Autodesk Inventor part; units mm, degrees
ref_plane "Work Plane5" through (0, -10, 0) normal (0, 1, 0) x (-1, 0, 0)
ref_plane "YZ Plane" through (0, 0, 0) normal (1, 0, 0) x (0, 1, 0)
ref_plane "XY Plane" through (0, 0, 0) normal (0, 0, 1) x (1, 0, 0)
sketch "Sketch1" plane through (0, 0, 0) normal (0, 0, 1) x (1, 0, 0)
  line L0 (-3.9007, 3.9007) -> (3.9007, 3.9007)
  line L1 (3.9007, 3.9007) -> (3.9007, -3.9007)
  line L2 (3.9007, -3.9007) -> (-3.9007, -3.9007)
  line L3 (-3.9007, -3.9007) -> (-3.9007, 3.9007)
  line L4 (0, 3.9007) -> (0, -3.9007) construction
  line L5 (-3.9007, 0) -> (3.9007, 0) construction
  circle A0 centre (0, 0) radius 2.1
  line L6 (0, 0) -> (-16.1173, 16.1173) construction
  line L7 (0, 0) -> (22.7933, 0) construction
  line L8 (-2.84, 3.9007) -> (-5.4993, 6.56)
  line L9 (-5.4993, 6.56) -> (-5.4993, 8.2)
  line L10 (-5.4993, 8.2) -> (-2.84, 8.2)
  line L11 (-2.84, 8.2) -> (-4.64, 10)
  line L12 (-4.64, 10) -> (-10, 10)
  line L13 (-10, 10) -> (-10, 4.64)
  line L14 (-10, 4.64) -> (-8.2, 2.84)
  line L15 (-8.2, 2.84) -> (-8.2, 5.4993)
  line L16 (-8.2, 5.4993) -> (-6.56, 5.4993)
  line L17 (-6.56, 5.4993) -> (-3.9007, 2.84)
  line L18 (-3.9007, 2.84) -> (-11.3102, 2.84) construction
  line L19 (-2.84, 3.9007) -> (-3.9007, 3.9007)
  line L20 (-3.9007, 2.84) -> (-3.9007, 3.9007)
  line L21 (-3.9007, -2.84) -> (-6.56, -5.4993)
  line L22 (-6.56, -5.4993) -> (-8.2, -5.4993)
  line L23 (-8.2, -5.4993) -> (-8.2, -2.84)
  line L24 (-8.2, -2.84) -> (-10, -4.64)
  line L25 (-10, -4.64) -> (-10, -10)
  line L26 (-10, -10) -> (-4.64, -10)
  line L27 (-4.64, -10) -> (-2.84, -8.2)
  line L28 (-2.84, -8.2) -> (-5.4993, -8.2)
  line L29 (-5.4993, -8.2) -> (-5.4993, -6.56)
  line L30 (-5.4993, -6.56) -> (-2.84, -3.9007)
  line L31 (-3.9007, -2.84) -> (-3.9007, -3.9007)
  line L32 (-2.84, -3.9007) -> (-3.9007, -3.9007)
  line L33 (2.84, -3.9007) -> (5.4993, -6.56)
  line L34 (5.4993, -6.56) -> (5.4993, -8.2)
  line L35 (5.4993, -8.2) -> (2.84, -8.2)
  line L36 (2.84, -8.2) -> (4.64, -10)
  line L37 (4.64, -10) -> (10, -10)
  line L38 (10, -10) -> (10, -4.64)
  line L39 (10, -4.64) -> (8.2, -2.84)
  line L40 (8.2, -2.84) -> (8.2, -5.4993)
  line L41 (8.2, -5.4993) -> (6.56, -5.4993)
  line L42 (6.56, -5.4993) -> (3.9007, -2.84)
  line L43 (2.84, -3.9007) -> (3.9007, -3.9007)
  line L44 (3.9007, -2.84) -> (3.9007, -3.9007)
  line L45 (3.9007, 2.84) -> (6.56, 5.4993)
  line L46 (6.56, 5.4993) -> (8.2, 5.4993)
  line L47 (8.2, 5.4993) -> (8.2, 2.84)
  line L48 (8.2, 2.84) -> (10, 4.64)
  line L49 (10, 4.64) -> (10, 10)
  line L50 (10, 10) -> (4.64, 10)
  line L51 (4.64, 10) -> (2.84, 8.2)
  line L52 (2.84, 8.2) -> (5.4993, 8.2)
  line L53 (5.4993, 8.2) -> (5.4993, 6.56)
  line L54 (5.4993, 6.56) -> (2.84, 3.9007)
  line L55 (3.9007, 2.84) -> (3.9007, 3.9007)
  line L56 (2.84, 3.9007) -> (3.9007, 3.9007)
  dimension "d7" = 4.2
  dimension "d8" = 135
  dimension "d9" = 1.5
  dimension "d10" = 1.64
  dimension "d11" = 1.8
  dimension "d12" = 2.84
  dimension "d13" = 10
  dimension "d16" = 360
extrude "Extrusion1" add sketch "Sketch1" along normal blind 150
pattern_linear "Rectangular Pattern1" count 2 spacing 20 along (0, -1, 0) of "Extrusion1"
sketch "Sketch2" plane through (0, 0, 150) normal (0, 0, 1) x (1, 0, 0)
  line L0 (8.2, -2.84) -> (8.2, -5.4993)
  line L1 (8.2, -5.4993) -> (6.56, -5.4993)
  line L2 (-6.56, -5.4993) -> (-8.2, -5.4993)
  line L3 (-8.2, -5.4993) -> (-8.2, -2.84)
  line L4 (-8.2, -14.5007) -> (-6.56, -14.5007)
  line L5 (6.56, -14.5007) -> (8.2, -14.5007)
  line L6 (5.4993, -11.8) -> (5.4993, -13.44)
  line L7 (5.4993, -13.44) -> (2.84, -16.0993)
  line L8 (-2.84, -16.0993) -> (-5.4993, -13.44)
  line L9 (-5.4993, -8.2) -> (-5.4993, -6.56)
  line L10 (-5.4993, -6.56) -> (-2.84, -3.9007)
  line L11 (2.84, -3.9007) -> (5.4993, -6.56)
  line L12 (2.84, -8.2) -> (4.64, -10)
  line L13 (-8.2, -6.9993) -> (-5.9387, -6.9993)
  line L14 (-5.9387, -6.9993) -> (-4.1231, -5.1837)
  line L15 (-4.1231, -5.1837) -> (4.1231, -5.1837)
  line L16 (4.1231, -5.1837) -> (5.9387, -6.9993)
  line L17 (5.9387, -6.9993) -> (8.2, -6.9993)
  line L18 (8.2, -6.9993) -> (8.2, -13.0007)
  line L19 (8.2, -13.0007) -> (5.9387, -13.0007)
  line L20 (5.9387, -13.0007) -> (4.2461, -14.6932)
  line L21 (4.2461, -14.6932) -> (-4.2461, -14.6932)
  line L22 (-4.2461, -14.6932) -> (-5.9387, -13.0007)
  line L23 (-5.9387, -13.0007) -> (-8.2, -13.0007)
  line L24 (-8.2, -13.0007) -> (-8.2, -6.9993)
  dimension "d23" = 1.5
  dimension "d24" = 1.5
  dimension "d25" = 1.5
  dimension "d26" = 1.5
extrude "Extrusion2" cut sketch "Sketch2" against normal up to next
ref_plane "Work Plane5" through (0, -10, 0) normal (0, 1, 0) x (-1, 0, 0)
equation "\"d24\" = d23"
equation "\"d25\" = d23"
equation "\"d26\" = d23"
properties part number "20x40x597mm" material "Aluminum 6061"
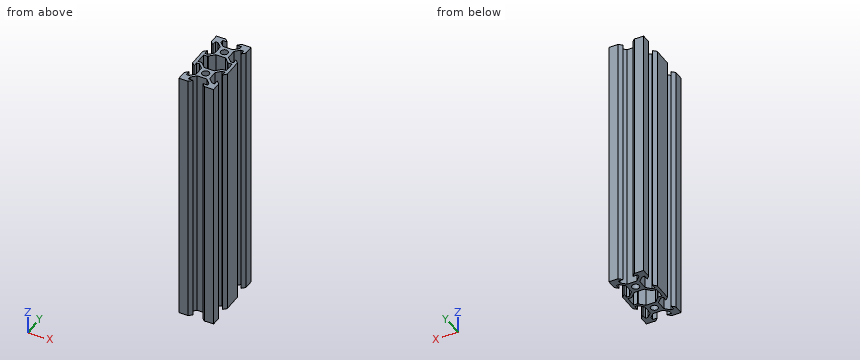
The listing builds one solid part. Answer for the finished solid, in the listing's coordinates (mm). Round coordinates to 2 decimals unless told otherwise and drop trailing zeros. Order: outer loops, then holes, each group sorted by start corner. A loop starts at its lowest first (then second) coordinate and runs counter-clockwise, first axis right, second up. Notation, with made-up numbers: (-27.5, 28) -> (20.5, 28) arc R32 cw to (20.5, 64) -> close; hole circle Ø3 at (22, 85.25). An arc over 180 degrees is marked (long way). Write each question's results on one line, items separated by ' | '. Start each with the question number.
Q1. Each of these flat-tipped pins is pushed along its axis until it touches: pin 1 (3 mm diameter, centred on y = -21.5, z = 109.5, fed in from +X); pin 2 (6 mm diameter, centred on x = -1.5, z = 107.5, fed in from +Y); pin 3 (1.3 mm diameter, centred on x = 3.5, z = 79.5, fed in from +Y). Where does it stop, or does it pass through?
Q2. Find section A-A (y = 0). Determine the outline of the cut face in (x, z), then the cut area to 3 significant figures.
Q3. Straight lines are drawn through the part: probe 1 along Y at (x, z) = (0, 49); probe 2 along Y at (x, z) = (-6.75, 142.5); probe 3 along Y at (x, z) = (4.5, 78). For each, find the intervals that lie inside material, in ascending order. Write a range as from..to.
Q4. Find section B-B (x = 0). Determine the outline of the cut face in (y, z).
Q5. Find section C-C (z = 120). Give the number of separate pieces and of enclosed holes in the cut face, then the cut area to 3 significant figures.
Worked answers:
1) pin 1: stops at x = 8.36 | pin 2: stops at y = 9.86 | pin 3: stops at y = 9.51
2) outline: (-3.9, 0) -> (-2.1, 0) -> (-2.1, 150) -> (-3.9, 150) -> close; (2.1, 0) -> (3.9, 0) -> (3.9, 150) -> (2.1, 150) -> close | area: 540 mm2
3) probe 1: y = -23.9..-22.1, -17.9..-16.1, -3.9..-2.1, 2.1..3.9 | probe 2: y = -30..-25.5, -14.5..-13, -7..-5.5, 5.5..10 | probe 3: y = -29.86..-28.2, -25.56..-23.44, -16.56..-14.44, -5.56..-3.44, 3.44..5.56, 8.2..9.86
4) outline: (-23.9, 0) -> (-22.1, 0) -> (-22.1, 150) -> (-23.9, 150) -> close; (-17.9, 0) -> (-16.1, 0) -> (-16.1, 150) -> (-17.9, 150) -> close; (-3.9, 0) -> (-2.1, 0) -> (-2.1, 150) -> (-3.9, 150) -> close; (2.1, 0) -> (3.9, 0) -> (3.9, 150) -> (2.1, 150) -> close
5) separate pieces: 1 | enclosed holes: 3 | area: 297 mm2
